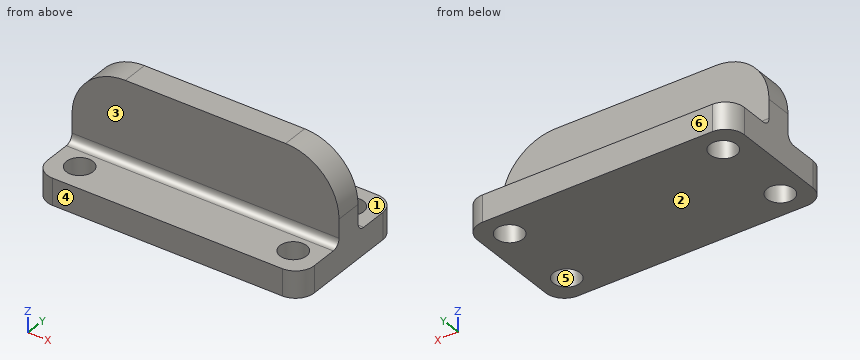
```python
from build123d import *

# Parameters (mm, degrees)
SKETCH_W     = 100
SKETCH_H     = 50
PAD_DEPTH    = 10
SKETCH001_W  = 100
SKETCH001_H  = 10
PAD001_DEPTH = 30
SKETCH002_R  = 5
POCKET_DEPTH = 10.001
FILLET_R     = 20
FILLET001_R  = 7
FILLET002_R  = 3


with BuildPart() as part:
    # Sketch → Pad (new body)
    with BuildSketch(Plane.XY):
        with Locations((50, 25)):
            Rectangle(SKETCH_W, SKETCH_H)
    extrude(amount=PAD_DEPTH)

    # Sketch001 (on Face6 of Pad) → Pad001 (join)
    with BuildSketch(Plane.XY.offset(10)):
        with Locations((50, 25)):
            Rectangle(SKETCH001_W, SKETCH001_H)
    extrude(amount=PAD001_DEPTH)

    # Sketch002 (on Face5 of Pad001) → Pocket (cut, through all)
    with BuildSketch(Plane.XY.offset(10)):
        with Locations((10, 40)):
            Circle(SKETCH002_R)
        with Locations((90, 40)):
            Circle(SKETCH002_R)
        with Locations((10, 10)):
            Circle(SKETCH002_R)
        with Locations((90, 10)):
            Circle(SKETCH002_R)
    extrude(amount=-POCKET_DEPTH, mode=Mode.SUBTRACT)

    # Fillet
    fillet_edges = [part.edges().sort_by_distance(p)[0] for p in [
        (100, 25, 40),
        (0, 25, 40),
    ]]
    fillet(fillet_edges, radius=FILLET_R)

    # Fillet001
    fillet001_edges = [part.edges().sort_by_distance(p)[0] for p in [
        (100, 0, 5),
        (100, 50, 5),
        (0, 0, 5),
        (0, 50, 5),
    ]]
    fillet(fillet001_edges, radius=FILLET001_R)

    # Fillet002
    fillet002_edges = [part.edges().sort_by_distance(p)[0] for p in [
        (50, 20, 10),
        (50, 30, 10),
    ]]
    fillet(fillet002_edges, radius=FILLET002_R)


solid = part.part
```
Source: CAD feature listing. Evaluate the final solid. Frame: model axes, mm. Face numbers are marked on the shaded views. A direction names the side the tool comes from. Coordinates: 2 decimals unless noted, no trailing zeros. Loops run counter-clockwise (first coordinate to the right, second up) from the corner with the lowest first, then second, coordinate; pieces in that order, holes last. Notation, with made-up numbers: M 37.25,36 L 44.25,36 A7 ccw 44.25,44 Z; hole C -22.75,43 d8. An arc over 180 degrees is marked long. Use CSV: the item, a comma, the result in double quotes.
(1) Cut plane A-A on y = 10. Return loops of the section in (x, z).
Answers follow:
outline,"M 0,0 L 5,0 L 5,10 L 0,10 Z; M 15,0 L 85,0 L 85,10 L 15,10 Z; M 95,0 L 100,0 L 100,10 L 95,10 Z"
(2) Contact query for flat-ended pins moving along their axis: pin 1 (16 mm diameter, centred on x = 10, y = 10, fed in from -Z); pin 2 (10 mm diameter, centred on x = 48.5, z = 22, fed in from +Y); pin 3 (13 mm diameter, centred on x = 90, y = 10, fed in from +Z); pin 4 (8 mm diameter, centred on y = 31, z = 34.5, fed in from -X). Output: stop coordinate, or through.
Answers follow:
pin 1,"z = 0"
pin 2,"y = 30"
pin 3,"z = 10"
pin 4,"x = 3.06"
(3) Cut plane B-B on z = 9. Return loops of the section in (x, y), and give its area (3 significant figures).
Answers follow:
outline,"M 0,7 A7 ccw 7,0 L 93,0 A7 ccw 100,7 L 100,43 A7 ccw 93,50 L 7,50 A7 ccw 0,43 Z; hole C 10,10 d10; hole C 10,40 d10; hole C 90,10 d10; hole C 90,40 d10"
area,"4,640 mm²"
(4) Draft query along Y for the marked faces 4, 5 and 6. Return one class per face: pulls with the +Y half, pulls with the -Y half, needs draft (parallel to the pull), parting line crosses it, or undercut.
Answers follow:
face 4,"pulls with the -Y half"
face 5,"undercut"
face 6,"pulls with the +Y half"
(5) Line query: line 1 (Y direction, x = 90, z = 6); line 2 (Y direction, x = 28.5, z = 34.5); line 3 (Z direction, x = 39.5, y = 10.5). Output: solid intervals per line, ascending. Write a range as [from, to].
Answers follow:
line 1,"[0, 5], [15, 35], [45, 50]"
line 2,"[20, 30]"
line 3,"[0, 10]"
(6) Cut plane D-D on x = 30. Return loops of the section in (y, z), and give its area (3 significant figures).
Answers follow:
outline,"M 0,0 L 50,0 L 50,10 L 33,10 A3 cw 30,13 L 30,40 L 20,40 L 20,13 A3 cw 17,10 L 0,10 Z"
area,"804 mm²"
(7) Cut plane C-C on x = 90.5. Return loops of the section in (y, z), and give its area (3 significant figures).
Answers follow:
outline,"M 0,0 L 5.03,0 L 5.03,10 L 0,10 Z; M 14.97,0 L 35.03,0 L 35.03,10 L 33,10 A3 cw 30,13 L 30,37.02 L 20,37.02 L 20,13 A3 cw 17,10 L 14.97,10 Z; M 44.97,0 L 50,0 L 50,10 L 44.97,10 Z"
area,"575 mm²"
(8) Reachability of the marked faces 1, 2 and 3 from +Z, -Z, +X, -X, +Y, -Y: full face, straight path, thin tool, end or side. Return the list, or none.
Answers follow:
face 1,"+Z, +X, -X, +Y"
face 2,"-Z, +X, -X, +Y, -Y"
face 3,"+Z, +X, -X, -Y"
